Verification items for the finished model (mm, model axes). Face numbers are marked on the shaded views. A direction names the side the tool comes from. Round coordinates to 2 decimals unless told otherwise and drop trailing zeros. Order: outer loops, then holes, each group sorted by start corner. A loop starts at its lowest first (then second) coordinate and runs counter-clockwise, first axis right, second up. Notation, with made-up numbers: (-21, 59) -> (0, 59) arc R23 ccw to (0, 96) -> close; hole circle Ø3 at (21, 73). An arc over 180 degrees is marked (long way). Put each result on its own line as item: value.
```python
from build123d import *

# Parameters (mm, degrees)
F0_R     = 5
F0_W     = 15.4567654431
F0_H     = 37.5
F1_DEPTH = 2.5
F3_DEPTH = 37.501
F2_R     = 3
F2_R_2   = 2.5
F4_DEPTH = 37.5


with BuildPart() as f1:
    # F0 (on Top) → F1 (new body)
    with BuildSketch(Plane.XY):
        with BuildLine():
            Line((0, 75), (0, 0))
            Line((0, 0), (20, 0))
            Line((20, 0), (20, 37.5))
            Line((20, 37.5), (20, 75))
            ThreePointArc((20, 75), (10, 65), (0, 75))
        make_face()
        with Locations((10, 11.628289707)):
            Circle(F0_R, mode=Mode.SUBTRACT)
        with Locations((27.7283827215, 18.75)):
            Rectangle(F0_W, F0_H)
        with BuildLine():
            ThreePointArc((20, 75), (10, 85), (0, 75))
            Line((0, 75), (5, 75))
            ThreePointArc((5, 75), (10, 80), (15, 75))
            Line((15, 75), (20, 75))
        make_face()
        with BuildLine():
            Line((5, 75), (0, 75))
            ThreePointArc((0, 75), (10, 65), (20, 75))
            Line((20, 75), (15, 75))
            ThreePointArc((15, 75), (10, 70), (5, 75))
        make_face()
    extrude(amount=F1_DEPTH)

    # F2 (on face) → F3 (cut, through all)
    with BuildSketch(Plane(origin=(0, 37.5, 0), x_dir=(-1, 0, 0), z_dir=(0, 1, 0))):
        with BuildLine():
            ThreePointArc((-32.9567654431, 1.25), (-33.0419508774, 1.8970476128), (-33.2917019336, 2.5))
            Line((-33.2917019336, 2.5), (-35.4567654431, 2.5))
            Line((-35.4567654431, 2.5), (-35.4567654431, 0))
            Line((-35.4567654431, 0), (-33.2917019336, 0))
            ThreePointArc((-33.2917019336, 0), (-33.0419508774, 0.6029523872), (-32.9567654431, 1.25))
        make_face()
    extrude(amount=-F3_DEPTH, mode=Mode.SUBTRACT)

    # F2 (on face) → F4 (join)
    with BuildSketch(Plane(origin=(0, 37.5, 0), x_dir=(-1, 0, 0), z_dir=(0, 1, 0))):
        with Locations((-35.4567654431, 1.25)):
            Circle(F2_R)
        with Locations((-35.4567654431, 1.25)):
            Circle(F2_R_2, mode=Mode.SUBTRACT)
    extrude(amount=-F4_DEPTH)


solid = f1.part
```
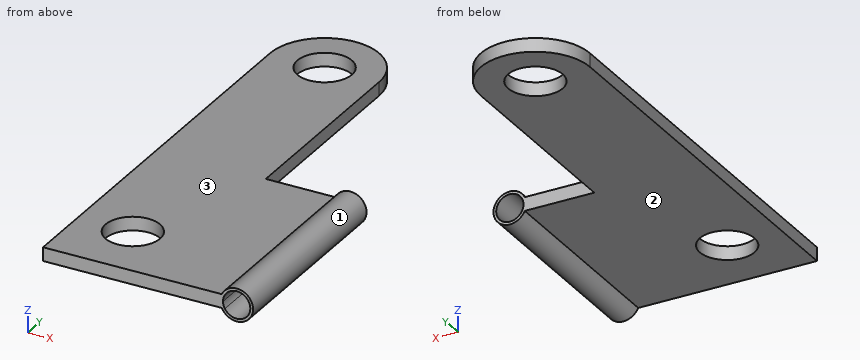
Item 1: Sectioned sample at C-C, the plane y = 55. Record the boundary of the cut face in (x, z), then the cut area to 3 significant figures.
Geometry check:
outline: (0, 0) -> (20, 0) -> (20, 2.5) -> (0, 2.5) -> close
area: 50.0 mm2
Item 2: Sectioned sample at A-A, the plane x = 10. Record the boundary of the cut face in (y, z).
Geometry check:
outline: (0, 0) -> (6.63, 0) -> (6.63, 2.5) -> (0, 2.5) -> close; (16.63, 0) -> (70, 0) -> (70, 2.5) -> (16.63, 2.5) -> close; (80, 0) -> (85, 0) -> (85, 2.5) -> (80, 2.5) -> close
Item 3: Material ranges on line 1 along X through (y, z) = (33, 1.25); line 2 along X through (y, z) = (8, 0.65); line 3 along Z through (x, y) = (6, 43.5), recorded low to high.
Geometry check:
line 1: 0 to 32.96, 37.96 to 38.46
line 2: 0 to 6.56, 13.44 to 33.03, 37.88 to 38.4
line 3: 0 to 2.5
Item 4: Sectioned sample at D-D, the plane x = 22.5. Record the boundary of the cut face in (y, z), then the cut area to 4 significant figures.
Geometry check:
outline: (0, 0) -> (37.5, 0) -> (37.5, 2.5) -> (0, 2.5) -> close
area: 93.75 mm2
Item 5: Sectioned sample at B-B, the plane y = 23. Record the boundary of the cut face in (x, z).
Geometry check:
outline: (0, 0) -> (32.73, 0) arc R3 ccw (long way) to (32.73, 2.5) -> (0, 2.5) -> close; hole circle Ø5 at (35.46, 1.25)
Item 6: Depth check by flat-ended pin: pin 1 Ø6 at (x, y) = (10, 75) entering from +Z; pin 2 Ø6 at (x, y) = (28, 40) entering from -Z; pin 3 Ø6 at (x, y) = (19.5, 73.5) entering from +Z; pin 4 Ø1.2 at (y, z) = (50.5, 1) entering from +X. Enter the tip coordinate at first touch or a pass-through.
Geometry check:
pin 1: through
pin 2: z = 0
pin 3: z = 2.5
pin 4: x = 20
Item 7: Tool access check on the marked faces 1, 2 and 3. Record the directions out of +Z, -Z, +X, -X, +Y, -Y that give a thin tool (end or side, any length) a straight path to the whole face; none if there is none.
Geometry check:
face 1: +Y, -Y
face 2: -Z, -X, +Y, -Y
face 3: +Z, -X, +Y, -Y
